Could you check a few things on this model? Use its own coordinates, in mm. Face numbers are marked on the shaded views. A direction names the side the tool comes from. Coordinates: 2 decimals unless noted, no trailing zeros. Loops run counter-clockwise (first coordinate to the right, second up) from the corner with the lowest first, then second, coordinate; pieces in that order, holes last. Notation, with made-up numbers: (-15, -6.75) - (28, -6.75) arc R36 cw to (28, 31.25) - close; hole circle Ø8 at (83.25, 56). An arc over 180 degrees is marked (long way). One line per question, with ' | ' between items. Start each with the question number.
1. We'd pull the mould along Z, two halves only. Please class the marked faces 1, 2, 3 and 4: pulls with the +Z half, pulls with the -Z half, needs draft (parallel to the pull), parting line crosses it, or undercut.
2. I want a section at C-C, the plane z = -2. Write out the boundary of the cut face in (x, y).
3. Please list where these lines run through material, in increasing order: L1, parallel to X at y = -7.75, z = 0.25; L2, parallel to Y at x = 5, z = -3.5; L3, parallel to X at y = -18, z = 1. Write a range as [from, to].
4. I'm going to push flat-ended pins straight in: P1, Ø9, axis at x = -0.5, y = -19.5, coming from the +Z side (3 decimals); P2, Ø1, axis at y = -10.5, z = -1.5, coming from the -X side; P3, Ø4, axis at y = -8.5, z = -5.5, coming from the +X side. Where does each tip first touch, or does it pass through?
5. Which directions (+Z, -Z, +X, -X, +Y, -Y) give clear straight access to the entire face, cutting with the end or side of a thin tool? Please do the marked faces 5, 6 and 7.
6. I want a section at B-B, the plane x = 0. Write out the boundary of the cut face in (y, z) (1 decimal).
from build123d import *

# Parameters (mm, degrees)
F0_R     = 9.525
F1_DEPTH = 25.4
F3_DEPTH = 25.401
F4_DEPTH = 12.7
F6_DEPTH = 12.7


with BuildPart() as f1:
    # F0 (on Front) → F1 (new body)
    with BuildSketch(Plane.XZ):
        Circle(F0_R)
    extrude(amount=F1_DEPTH)

    # F2 (on Front) → F3 (cut, through all)
    with BuildSketch(Plane.XZ):
        with BuildLine():
            ThreePointArc((4.7625, 0), (3.367596, 3.367596), (0, 4.7625))
            ThreePointArc((0, 4.7625), (-3.367596, 3.367596), (-4.7625, 0))
            ThreePointArc((-4.7625, 0), (-3.367596, -3.367596), (0, -4.7625))
            ThreePointArc((0, -4.7625), (3.367596, -3.367596), (4.7625, 0))
        make_face()
    extrude(amount=F3_DEPTH, mode=Mode.SUBTRACT)

    # F2 (on Front) → F4 (cut)
    with BuildSketch(Plane.XZ):
        with BuildLine():
            Line((4.7625, -4.7625), (4.7625, 0))
            ThreePointArc((4.7625, 0), (3.367596, -3.367596), (0, -4.7625))
            Line((0, -4.7625), (4.7625, -4.7625))
        make_face()
        with BuildLine():
            Line((4.7625, 4.7625), (0, 4.7625))
            ThreePointArc((0, 4.7625), (3.367596, 3.367596), (4.7625, 0))
            Line((4.7625, 0), (4.7625, 4.7625))
        make_face()
        with BuildLine():
            Line((0, 4.7625), (-4.7625, 4.7625))
            Line((-4.7625, 4.7625), (-4.7625, 0))
            ThreePointArc((-4.7625, 0), (-3.367596, 3.367596), (0, 4.7625))
        make_face()
        with BuildLine():
            ThreePointArc((0, -4.7625), (-3.367596, -3.367596), (-4.7625, 0))
            Line((-4.7625, 0), (-4.7625, -4.7625))
            Line((-4.7625, -4.7625), (0, -4.7625))
        make_face()
    extrude(amount=F4_DEPTH, mode=Mode.SUBTRACT)

    # F5 (on face) → F6 (cut)
    with BuildSketch(Plane.XZ.offset(25.4)):
        Polygon((4.1275, 7.14904), (-4.1275, 7.14904), (-8.255, 0), (-4.1275, -7.14904), (4.1275, -7.14904), (8.255, 0), align=None)
    extrude(amount=-F6_DEPTH, mode=Mode.SUBTRACT)


solid = f1.part
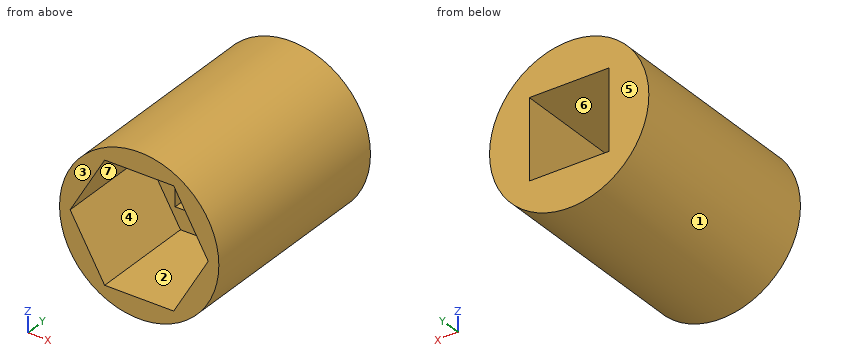
Results are:
1) face 1: parting line crosses it | face 2: undercut | face 3: needs draft | face 4: undercut
2) outline: (-9.31, -25.4) - (-7.1, -25.4) - (-7.1, -12.7) - (-4.76, -12.7) - (-4.76, 0) - (-9.31, 0) - close; (4.76, -12.7) - (7.1, -12.7) - (7.1, -25.4) - (9.31, -25.4) - (9.31, 0) - (4.76, 0) - close
3) L1: x = [-9.52, -4.76], [4.76, 9.52] | L2: y = [-12.7, 0] | L3: x = [-9.47, -7.68], [7.68, 9.47]
4) P1: stops at z = 9.525 | P2: stops at x = -9.47 | P3: stops at x = 8.86
5) face 5: +Z, -Z, +X, -X, +Y | face 6: +Y, -Y | face 7: -Y
6) outline: (-25.4, -9.5) - (0, -9.5) - (0, -4.8) - (-12.7, -4.8) - (-12.7, -7.1) - (-25.4, -7.1) - close; (-25.4, 7.1) - (-12.7, 7.1) - (-12.7, 4.8) - (0, 4.8) - (0, 9.5) - (-25.4, 9.5) - close
